Geometry: final body of the model. Coordinates: model frame, mm. A direction names the side the tool comes from. Give positions to 0.01 mm unless a question says otherwise; leave off trailing zeros. Loops run counter-clockwise (first coordinate to the right, second up) from the corner with the lowest first, then second, coordinate; pieces in that order, holes last.
1. Section B-B, the plane x = 0. Output: boundary loops of the cut face in (y, z) (1 decimal), then the cut area to 3 significant figures.
2. Section C-C, the plane y = 20.32. Output: boundary loops of the cut face in (x, z), then the cut area to 3 significant figures.
3. Section A-A, the plane x = -9. Output: boundary loops of the cut face in (y, z) (3 decimals), then the cut area to 3 significant figures.
4. Material intervals for line 1 along Y through (x, z) = (-13.75, 0.3) (3 decimals); line 2 along Y through (x, z) = (2.25, 0.35) (3 decimals); line 3 along X through (y, z) = (21, 0.75), sorted ascending.
5. Access query for faces 1 (the face through (3, -17.145, 1)), 2 (the face through (1.816, -43, 1)), 3 (the face through (-4, 4.445, 1)). Directions: +Z, -Z, +X, -X, +Y, -Y. A direction counts if a zero-diameter tool reaches every point of the face in a straight line with its end or side. Return the directions, or none.
6. Section D-D, the plane y = -0.5. Output: boundary loops of the cut face in (x, z), then the cut area to 3 significant figures.
7. Draft query along Y for faces 4 (the face through (-12, 16.383, 2)), 5 (the face through (3, -36.989, 1)), 6 (the face through (4.762, -33, 1)), 7 (the face through (-5.717, 17.288, 1.459)). Return one class per face: +Y half, -Y half, draft (parallel to the pull), parting line (faces both ways), or undercut.
8. First-contact query: P1, Ø0.8, axis at x = -4, z = 2, coming from the -Y side (3 decimals); P2, Ø1.3, axis at x = -10.63, y = 13.9, coming from the +Z side; P3, Ø0.9, axis at y = -2, z = 2, coming from the -X side; P4, Ø1.5, axis at y = -5, z = 1, coming from the +X side. Flat tips, straight axial feed; report the tip coordinate or a pass-through.
from build123d import *

# Parameters (mm, degrees)
SKETCH1_R             = 3.175
BOSS_EXTRUDE1_DEPTH   = 2.9591
SKETCH8_W             = 1.5875
SKETCH8_H             = 3.175
CUT_EXTRUDE4_DEPTH    = 50.215431564
SKETCH4_W             = 11.7348
SKETCH4_H             = 4.9657
BOSS_EXTRUDE2_DEPTH   = 2.9591
FILLET1_R             = 3.175
F_0_CLEARANCE_HOLE1_D = 1.397
F_4_CLEARANCE_HOLE1_D = 2.9464
BOSS_EXTRUDE3_START   = -2.9591
BOSS_EXTRUDE3_DEPTH   = 2.9591
FILLET2_R             = 6.35
CUT_EXTRUDE5_REACH    = 53.688
SKETCH12_R            = 4.7625


with BuildPart() as part:
    # Sketch1 → Boss-Extrude1 (new body)
    with BuildSketch(Plane.XY):
        with BuildLine():
            Line((4.7625, 33.02), (4.7625, -17.145))
            Line((4.7625, -17.145), (1.8161, -17.145))
            Line((1.8161, -17.145), (1.8161, -29.05125))
            Line((1.8161, -29.05125), (4.7625, -29.05125))
            Line((4.7625, -29.05125), (4.7625, -36.98875))
            Line((4.7625, -36.98875), (1.8161, -36.98875))
            Line((1.8161, -36.98875), (1.8161, -48.895))
            Line((1.8161, -48.895), (-3.175, -48.895))
            Line((-3.175, -48.895), (-3.175, -42.545))
            Line((-3.175, -42.545), (-4.7625, -42.545))
            Line((-4.7625, -42.545), (-4.7625, -23.495))
            Line((-4.7625, -23.495), (-3.175, -23.495))
            Line((-3.175, -23.495), (-3.175, -17.145))
            Line((-3.175, -17.145), (-4.7625, -17.145))
            Line((-4.7625, -17.145), (-4.7625, 33.02))
            ThreePointArc((-4.7625, 33.02), (0, 37.7825), (4.7625, 33.02))
        make_face()
        with Locations((0, 33.02)):
            Circle(SKETCH1_R, mode=Mode.SUBTRACT)
    extrude(amount=BOSS_EXTRUDE1_DEPTH)

    # Sketch8 → Cut-Extrude4 (cut, through all)
    with BuildSketch(Plane(origin=(0, 0, 0), x_dir=(-1, 0, 0), z_dir=(0, 0, -1))):
        with Locations((-3.96875, 6.0325)):
            Rectangle(SKETCH8_W, SKETCH8_H)
        with Locations((3.96875, 6.0325)):
            Rectangle(SKETCH8_W, SKETCH8_H)
    extrude(amount=-CUT_EXTRUDE4_DEPTH, mode=Mode.SUBTRACT)

    # Sketch4 → Boss-Extrude2 (add)
    with BuildSketch(Plane.XY.offset(2.9591)):
        with Locations((-10.6299, 13.90015)):
            Rectangle(SKETCH4_W, SKETCH4_H)
        with Locations((-10.6299, -14.66215)):
            Rectangle(SKETCH4_W, SKETCH4_H)
    extrude(amount=-BOSS_EXTRUDE2_DEPTH)

    # Fillet1
    fillet1_edges = [part.edges().sort_by_distance(p)[0] for p in [
        (-4.7625, 16.383, 1.47955),
    ]]
    fillet(fillet1_edges, radius=FILLET1_R)

    # #0 Clearance Hole1 (through all)
    with Locations(Plane(origin=(0, 0, 0), x_dir=(-1, 0, 0), z_dir=(0, 0, -1))):
        with Locations((10.6299, 13.90015), (10.6299, -14.66215)):
            Hole(F_0_CLEARANCE_HOLE1_D / 2)

    # #4 Clearance Hole1 (through all)
    with Locations(Plane.XY.offset(2.9591)):
        with Locations((0, 20.32)):
            Hole(F_4_CLEARANCE_HOLE1_D / 2)

    # Sketch11 → Boss-Extrude3 (add)
    with BuildSketch(Plane.XY.offset(2.9591).offset(BOSS_EXTRUDE3_START)):
        with BuildLine():
            Line((-6.35, 33.02), (-6.35, 26.67))
            Line((-6.35, 26.67), (-4.7625, 20.32))
            Line((-4.7625, 20.32), (-4.7625, 33.02))
            ThreePointArc((-4.7625, 33.02), (0, 37.7825), (4.7625, 33.02))
            Line((4.7625, 33.02), (4.7625, 20.32))
            Line((4.7625, 20.32), (6.35, 26.67))
            Line((6.35, 26.67), (6.35, 33.02))
            ThreePointArc((6.35, 33.02), (0, 39.37), (-6.35, 33.02))
        make_face()
    extrude(amount=BOSS_EXTRUDE3_DEPTH)

    # Fillet2
    # the kernel refuses this fillet: 6.35 mm, written as the material it adds along each edge
    with BuildSketch(Plane(origin=(4.7625, 20.32, 0), x_dir=(0, -1, 0), z_dir=(0, 0, 1))) as fillet2_piece_1:
        with BuildLine():
            CenterArc((FILLET2_R * 0.123105625618, FILLET2_R), FILLET2_R, 255.963756532, 14.036243468)
            Line((-FILLET2_R * 0.119429999419, FILLET2_R * 0.0298574998547), (0, 0))
            Line((0, 0), (FILLET2_R * 0.123105625618, 0))
        make_face()
    extrude(amount=2.9591)
    with BuildSketch(Plane(origin=(-4.7625, 20.32, 0), x_dir=(-8.465505129601726e-05, -0.9999999964167612, 0), z_dir=(0, 0, 1))) as fillet2_piece_2_section:
        with BuildLine():
            CenterArc((0.78250954, -6.349870963), FILLET2_R, 90.365265554, 13.675828291)
            Line((-0.758113183, -0.189596486), (-0.912175455, 0.426430961))
            Line((-0.912175455, 0.426430961), (-0.154062272, 0.616027448))
            Line((-0.154062272, 0.616027448), (-5.3756e-05, 0.634999998))
            ThreePointArc((-5.3756e-05, 0.634999998), (0.761946241, 0.635064505), (0.737979862, 0.634987096))
            Line((0.737979862, 0.634987096), (0.742028014, 0))
        make_face()
    fillet2_piece_2 = extrude(amount=2.9591, mode=Mode.PRIVATE)
    fillet2_piece_2 = split(fillet2_piece_2, bisect_by=Plane(origin=(-4.799885723, 7.62, 1.47955), z_dir=(0, 1, 0)), keep=Keep.TOP, mode=Mode.PRIVATE)
    fillet2_piece_2 = split(fillet2_piece_2, bisect_by=Plane(origin=(-3.175, 20.335301711, 1.47955), z_dir=(-1, 0, 0)), keep=Keep.TOP, mode=Mode.PRIVATE)
    add(fillet2_piece_2)
    # the kernel refuses this fillet: 6.35 mm, written as the material it takes off along each edge
    with BuildSketch(Plane(origin=(6.35, 26.67, -1.954301807), x_dir=(0, 1, 0), z_dir=(0, 0, 1))) as fillet2_2_piece_1:
        with BuildLine():
            CenterArc((FILLET2_R * 0.123105625618, FILLET2_R), FILLET2_R, 255.963756532, 14.036243468)
            Line((-FILLET2_R * 0.119429999419, FILLET2_R * 0.0298574998547), (0, 0))
            Line((0, 0), (FILLET2_R * 0.123105625618, 0))
        make_face()
    extrude(amount=6.867703613, mode=Mode.SUBTRACT)
    with BuildSketch(Plane(origin=(-6.35, 26.67, -1.954301807), x_dir=(0, 1, 0), z_dir=(0, 0, 1))) as fillet2_2_piece_2:
        with BuildLine():
            CenterArc((FILLET2_R * 0.123105625618, -FILLET2_R), FILLET2_R, 90, 14.036243468)
            Line((-FILLET2_R * 0.119429999419, -FILLET2_R * 0.0298574998547), (0, 0))
            Line((0, 0), (FILLET2_R * 0.123105625618, 0))
        make_face()
    extrude(amount=6.867703613, mode=Mode.SUBTRACT)

    # Sketch12 → Cut-Extrude5 (cut, up to next)
    with BuildSketch(Plane.XY.offset(2.9591), mode=Mode.PRIVATE) as cut_extrude5_sk1:
        with Locations((0, 33.02)):
            Circle(SKETCH12_R)
    cut_extrude5_tool1 = extrude(cut_extrude5_sk1.sketch, amount=-CUT_EXTRUDE5_REACH, mode=Mode.PRIVATE) & part.part
    add(cut_extrude5_tool1.solids().sort_by_distance((0, 33.02, 2.9591))[0], mode=Mode.SUBTRACT)


solid = part.part
Answers below:
1. outline: (-48.9, 0) - (18.8, 0) - (18.8, 3) - (-48.9, 3) - close; (21.8, 0) - (28.3, 0) - (28.3, 3) - (21.8, 3) - close; (37.8, 0) - (39.4, 0) - (39.4, 3) - (37.8, 3) - close
1. area: 224 mm2
2. outline: (-4.81, 0) - (-1.47, 0) - (-1.47, 2.96) - (-4.81, 2.96) - close; (1.47, 0) - (4.81, 0) - (4.81, 2.96) - (1.47, 2.96) - close
2. area: 19.8 mm2
3. outline: (-17.145, 0) - (-12.179, 0) - (-12.179, 2.959) - (-17.145, 2.959) - close; (11.417, 0) - (16.383, 0) - (16.383, 2.959) - (11.417, 2.959) - close
3. area: 29.4 mm2
4. line 1: y = -17.145 to -12.179, 11.417 to 16.383
4. line 2: y = -36.989 to -29.051, -17.145 to 28.823, 37.217 to 38.958
4. line 3: x = -4.93 to -1.31, 1.31 to 4.93
5. face 1: +Z, -Z, +X
5. face 2: +Z, -Z, +X, -Y
5. face 3: +Z, -Z, -X
6. outline: (-4.76, 0) - (4.76, 0) - (4.76, 2.96) - (-4.76, 2.96) - close
6. area: 28.2 mm2
7. face 4: +Y half
7. face 5: -Y half
7. face 6: draft
7. face 7: undercut
8. P1: stops at y = -42.545
8. P2: passes through
8. P3: stops at x = -4.76
8. P4: stops at x = 4.76
